Autodesk Fusion 360 part; units mm, degrees
sketch "Sketch1" plane through (0, 0, 0) normal (1, 0, 0) x (0, 1, 0)
  line L0 (0, 0) -> (0, 50)
  line L1 (0, 0) -> (125, 0)
  line L2 (125, 0) -> (150, 0)
  line L3 (150, 0) -> (150, 50)
  line L4 (0, 50) -> (50, 150)
  line L5 (50, 150) -> (100, 150)
  line L6 (100, 150) -> (150, 50)
  circle A0 centre (75, 125) radius 10
extrude "Extrude1" add sketch "Sketch1" along normal blind 5 makes body 1
ref_plane "WorkPlane1" through (275, 75, 75) normal (1, 0, 0) x (0, 1, 0)
sketch "Sketch2" plane through (275, 75, 75) normal (1, 0, 0) x (0, 1, 0)
  line L0 (-75, -75) -> (-75, -25)
  line L1 (-75, -25) -> (-25, 75)
  line L2 (-25, 75) -> (25, 75)
  line L3 (25, 75) -> (75, -25)
  line L4 (75, -25) -> (75, -75)
  line L5 (75, -75) -> (-75, -75)
  circle A0 centre (0, 50) radius 10
extrude "Extrude2" add sketch "Sketch2" along normal blind 5 separate body makes body 2
sketch "Sketch3" plane through (0, 0, 0) normal (0, 1, 0) x (1, 0, 0)
  line L0 (5, 0) -> (275, 0)
  line L1 (275, 0) -> (275, -50)
  line L2 (275, -50) -> (235, -50)
  line L3 (235, -50) -> (235, -50)
  line L4 (220, -35) -> (60, -35)
  line L5 (45, -50) -> (45, -50)
  line L6 (45, -50) -> (5, -50)
  line L7 (5, -50) -> (5, 0)
  arc A0 (60, -35) -> (45, -50) centre (60, -50) ccw
  arc A1 (235, -50) -> (220, -35) centre (220, -50) ccw
  dimension "d6" = 15
  dimension "d7" = 15
extrude "Extrude3" add sketch "Sketch3" along normal blind 5 bodies 1 2
ref_plane "WorkPlane2" through (0, 150, 0) normal (0, 1, 0) x (0, 0, 1)
sketch "Sketch4" plane through (0, 150, 0) normal (0, 1, 0) x (1, 0, 0)
  line L0 (5, -50) -> (5, 0)
  line L1 (5, 0) -> (275, 0)
  line L2 (275, 0) -> (275, -50)
  line L3 (275, -50) -> (235, -50)
  line L4 (235, -50) -> (235, -50)
  line L5 (220, -35) -> (60, -35)
  line L6 (45, -50) -> (45, -50)
  line L7 (45, -50) -> (5, -50)
  arc A0 (60, -35) -> (45, -50) centre (60, -50) ccw
  arc A1 (235, -50) -> (220, -35) centre (220, -50) ccw
  dimension "d11" = 15
  dimension "d12" = 15
extrude "Extrude4" add sketch "Sketch4" against normal blind 5 bodies 1
sketch "Sketch5" plane through (0, 0, 0) normal (0, 0, 1) x (1, 0, 0)
  line L0 (0, 150) -> (0, 0)
  line L1 (0, 0) -> (280, 0)
  line L2 (280, 0) -> (280, 150)
  line L3 (280, 150) -> (0, 150)
extrude "Extrude5" add sketch "Sketch5" against normal blind 10 bodies 1
sketch "Sketch6" plane through (280, 0, 0) normal (1, 0, 0) x (0, 1, 0)
  circle A0 centre (75, 125) radius 10
  line L0 (150, -10) -> (150, 50)
  line L1 (150, 50) -> (100, 150)
  line L2 (100, 150) -> (50, 150)
  line L3 (50, 150) -> (0, 50)
  line L4 (0, 50) -> (0, -10)
  line L5 (0, -10) -> (150, -10)
  circle A1 centre (75, 125) radius 10
extrude "Extrude6" add sketch "Sketch6" against normal blind 280 contours A0 A1 bodies 1
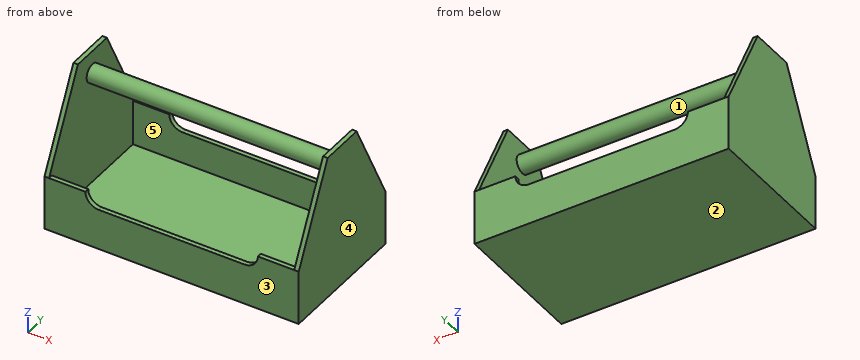
CAD build for the part. Positions are in the model's coordinates, mm. Face numbers are marked on the shaded views. A direction names the side the tool comes from. Give positions to 0.01 mm unless a question says otherwise; leave off trailing zeros. Order: outer loops, then holes, each group sorted by start corner. A loop starts at its lowest first (then second) coordinate and runs counter-clockwise, first axis right, second up.
(1) Flat gauge pins, fed straight in: pin 1 (2.5 mm diameter, centred on x = 125, y = 1.5, fed in from +Z); pin 2 (2.5 mm diameter, centred on x = 245.5, y = 3, fed in from +Z). Where does each tip first touch, or does it go through?
(2) Drill centre lines: L1, parallel to Y at x = 39, z = 22; L2, parallel to X at y = 110.5, z = 83.5; L3, parallel to Z at x = 228, y = 75. Where is each one in solid material? Low to high.
(3) Saw through at C-C, the plane y = 41.5. Give the cut face in (x, z), then the cut area to 3 significant figures.
(4) Tool access for the marked faces 4 and 5: list every direction of +Z, -Z, +X, -X, +Y, -Y with a clear straight run to the whole face (end or side of a thin tool).
(5) Mould opens along Z. For the marked faces 1, 2 and 3 say: released by +Z, released by -Z, zero draft, split by the parting line, or undercut.
(6) Saw through at B-B, the plane z = 58.5. Give the cut face in (x, y).
(7) Saw through at D-D, the plane z = 9.5. Give the cut face in (x, y), then the cut area to 3 significant figures.
(8) Saw through at A-A, the plane x = 24. Give the cut face in (y, z), then the cut area to 3 significant figures.
Results found:
1. pin 1: stops at z = 35
1. pin 2: stops at z = 50
2. L1: y = 0 to 5, 145 to 150
2. L2: x = 0 to 5, 275 to 280
2. L3: z = -10 to 0, 115 to 135
3. outline: (0, -10) - (280, -10) - (280, 133) - (275, 133) - (275, 0) - (5, 0) - (5, 133) - (0, 133) - close
3. area: 4,130 mm2
4. face 4: +Z, -Z, +X, +Y, -Y
4. face 5: +Z
5. face 1: undercut
5. face 2: released by -Z
5. face 3: zero draft
6. outline: (0, 4.25) - (5, 4.25) - (5, 145.75) - (0, 145.75) - close; (275, 4.25) - (280, 4.25) - (280, 145.75) - (275, 145.75) - close
7. outline: (0, 0) - (280, 0) - (280, 150) - (0, 150) - close; hole (5, 5) - (275, 5) - (275, 145) - (5, 145) - close
7. area: 4,200 mm2
8. outline: (0, -10) - (150, -10) - (150, 50) - (145, 50) - (145, 0) - (5, 0) - (5, 50) - (0, 50) - close; circle Ø20 at (75, 125)
8. area: 2,310 mm2
